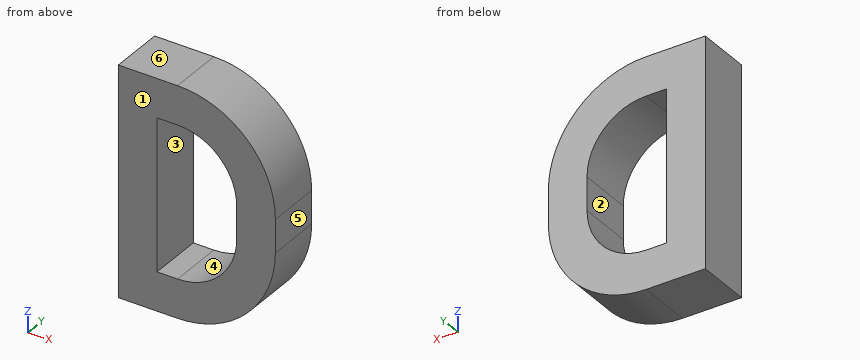
from build123d import *

# Parameters (mm, degrees)
F1_DEPTH = 12.7
F2_DEPTH = 12.7


with BuildPart() as f1:
    # F0 (on Front) → F1 (new body)
    with BuildSketch(Plane.XZ):
        with BuildLine():
            Line((-43.261304, 3.828095), (-52.208334, 3.828095))
            Line((-52.208334, 3.828095), (-52.208334, -22.648397))
            Line((-52.208334, -22.648397), (-38.501772, -22.648397))
            ThreePointArc((-38.501772, -22.648397), (-22.486937, -16.014835), (-15.853375, 0))
            Line((-15.853375, 0), (-15.853375, 3.828095))
            Line((-15.853375, 3.828095), (-24.800405, 3.828095))
            Line((-24.800405, 3.828095), (-24.800405, 0))
            ThreePointArc((-24.800405, 0), (-28.813443, -9.68833), (-38.501772, -13.701367))
            Line((-38.501772, -13.701367), (-43.261304, -13.701367))
            Line((-43.261304, -13.701367), (-43.261304, 3.828095))
        make_face()
    extrude(amount=F1_DEPTH)

    # F0 (on Front) → F2 (join)
    with BuildSketch(Plane.XZ):
        with BuildLine():
            Line((-38.501772, 30.304587), (-52.208334, 30.304587))
            Line((-52.208334, 30.304587), (-52.208334, 3.828095))
            Line((-52.208334, 3.828095), (-43.261304, 3.828095))
            Line((-43.261304, 3.828095), (-43.261304, 21.357557))
            Line((-43.261304, 21.357557), (-38.501772, 21.357557))
            ThreePointArc((-38.501772, 21.357557), (-28.813443, 17.34452), (-24.800405, 7.65619))
            Line((-24.800405, 7.65619), (-24.800405, 3.828095))
            Line((-24.800405, 3.828095), (-15.853375, 3.828095))
            Line((-15.853375, 3.828095), (-15.853375, 7.65619))
            ThreePointArc((-15.853375, 7.65619), (-22.486937, 23.671025), (-38.501772, 30.304587))
        make_face()
        with BuildLine():
            Line((-43.261304, 3.828095), (-52.208334, 3.828095))
            Line((-52.208334, 3.828095), (-52.208334, -22.648397))
            Line((-52.208334, -22.648397), (-38.501772, -22.648397))
            ThreePointArc((-38.501772, -22.648397), (-22.486937, -16.014835), (-15.853375, 0))
            Line((-15.853375, 0), (-15.853375, 3.828095))
            Line((-15.853375, 3.828095), (-24.800405, 3.828095))
            Line((-24.800405, 3.828095), (-24.800405, 0))
            ThreePointArc((-24.800405, 0), (-28.813443, -9.68833), (-38.501772, -13.701367))
            Line((-38.501772, -13.701367), (-43.261304, -13.701367))
            Line((-43.261304, -13.701367), (-43.261304, 3.828095))
        make_face()
    extrude(amount=F2_DEPTH)


solid = f1.part
The listing builds one solid part. Answer for the finished solid, in the listing's coordinates (mm). Face numbers are marked on the shaded views. A direction names the side the tool comes from. Give positions to 0.01 mm unless a question says otherwise; leave off trailing zeros. Write each loop counter-clockwise with the first axis right and the second up, starting at its lowest first coordinate (ties: lowest second). Pieces come first, ordered by that corner, then holes.
Item 1: Determine the mould class of the marked faces 3, 4, 5 and 6 for opening direction Z: released by +Z, released by -Z, zero draft, split by the parting line, or undercut.
Item 2: Section D-D, the plane x = -24 is taken. Write down the section's boundary in (y, z).
Item 3: Section C-C, the plane z = 7 is taken. Write down the section's boundary in (x, y), plus the area to 3 significant figures.
Item 4: Which of the six approach directions +Z, -Z, +X, -X, +Y, -Y give full straight-line access (tool end or side, diameter ignored) to the marked faces 1 and 2?
Item 5: Section B-B, the plane y = -4.5 is taken. Write down the section's boundary in (x, z).
Item 6: Section A-A, the plane x = -39.5 is taken. Write down the section's boundary in (y, z), plus the area to 3 significant figures.
Item 7: Flat-ended cylindrical pins translate along their axes: P1, Ø2, axis at x = -24.5, y = -9, coming from the +Z side; P2, Ø4, axis at y = -4, z = 12.5, coming from the +X side. Find the tip coordinate at first contact, or state that the pin passes through.
Item 8: Find the intervals of material crossed by line 1 along Z through (x, y) = (-40.5, -10.25); line 2 along X through (y, z) = (-8.25, 2); line 3 along Z through (x, y) = (-38, -11.5), in increasing order.
Completed:
1. face 3: undercut
1. face 4: undercut
1. face 5: zero draft
1. face 6: released by +Z
2. outline: (-12.7, -17.4) - (0, -17.4) - (0, 25.05) - (-12.7, 25.05) - close
3. outline: (-52.21, -12.7) - (-43.26, -12.7) - (-43.26, 0) - (-52.21, 0) - close; (-24.8, -12.7) - (-15.85, -12.7) - (-15.85, 0) - (-24.8, 0) - close
3. area: 227 mm2
4. face 1: +Z, -Z, +X, -X, -Y
4. face 2: +Y, -Y
5. outline: (-52.21, -22.65) - (-38.5, -22.65) arc R22.65 ccw to (-15.85, 0) - (-15.85, 7.66) arc R22.65 ccw to (-38.5, 30.3) - (-52.21, 30.3) - close; hole (-43.26, -13.7) - (-38.5, -13.7) arc R13.7 ccw to (-24.8, 0) - (-24.8, 7.66) arc R13.7 ccw to (-38.5, 21.36) - (-43.26, 21.36) - close
6. outline: (-12.7, -22.65) - (0, -22.65) - (0, -13.7) - (-12.7, -13.7) - close; (-12.7, 21.36) - (0, 21.36) - (0, 30.3) - (-12.7, 30.3) - close
6. area: 227 mm2
7. P1: stops at z = 26.2
7. P2: stops at x = -16.03
8. line 1: z = -22.65 to -13.7, 21.36 to 30.3
8. line 2: x = -52.21 to -43.26, -24.8 to -15.85
8. line 3: z = -22.64 to -13.69, 21.35 to 30.3
